```python
from build123d import *
from OCP.BRepFilletAPI import BRepFilletAPI_MakeChamfer

# Parameters (mm, degrees)
RESSALTO_EXTRUS_O2_DEPTH = 13
ESBO_O3_R                = 9.325
CORTE_EXTRUS_O1_DEPTH    = 27.211129951
ESBO_O4_W                = 8.746276247
ESBO_O4_H                = 4.85
CORTE_EXTRUS_O2_DEPTH    = 6.35
CHANFRO1_SIZE            = 2.5
CHANFRO1_SIZE2           = 1.443375673
CHANFRO2_SIZE            = 2
CHANFRO2_SIZE2           = 1.154700538
CHANFRO3_SIZE            = 2
CHANFRO3_SIZE2           = 1.154700538


with BuildPart() as part:
    # Esboço1 → Ressalto-extrusão2 (new body)
    with BuildSketch(Plane.XY):
        Polygon((0, 17.205038022), (-14.9, 8.602519011), (-14.9, -8.602519011), (0, -17.205038022), (14.9, -8.602519011), (14.9, 8.602519011), align=None)
    extrude(amount=RESSALTO_EXTRUS_O2_DEPTH)

    # Esboço3 → Corte-extrusão1 (cut, through all)
    with BuildSketch(Plane.XY.offset(13)):
        Circle(ESBO_O3_R)
    extrude(amount=-CORTE_EXTRUS_O1_DEPTH, mode=Mode.SUBTRACT)

    # Esboço4 → Corte-extrusão2 (cut)
    with BuildSketch(Plane.XY.offset(13)):
        with Locations((-10.526861876, 0)):
            Rectangle(ESBO_O4_W, ESBO_O4_H)
        Polygon((-5.349888396, 14.116278516), (-9.550111604, 11.691278516), (-5.176973481, 4.116781098), (-0.976750273, 6.541781098), align=None)
        Polygon((9.550111604, 11.691278516), (5.349888396, 14.116278516), (0.976750273, 6.541781098), (5.176973481, 4.116781098), align=None)
        with Locations((10.526861876, 0)):
            Rectangle(ESBO_O4_W, ESBO_O4_H)
        Polygon((5.349888396, -14.116278516), (9.550111604, -11.691278516), (5.176973481, -4.116781098), (0.976750273, -6.541781098), align=None)
        Polygon((-9.550111604, -11.691278516), (-5.349888396, -14.116278516), (-0.976750273, -6.541781098), (-5.176973481, -4.116781098), align=None)
    extrude(amount=-CORTE_EXTRUS_O2_DEPTH, mode=Mode.SUBTRACT)

    # Chanfro1: one chamfer whose edges measure the first distance from different faces: ONE call of the kernel's chamfer builder (chamfer() names one face for all edges)
    chanfro1_edges_1 = [part.edges().sort_by_distance(p)[0] for p in [
        (-14.9, 5.513759505, 13),
        (-14.9, -5.513759505, 13),
    ]]
    chanfro1_side_1 = [part.faces().sort_by_distance(p)[0] for p in [
        (-14.9, 0, 5.969058161),
    ]]
    chanfro1_edges_2 = [part.edges().sort_by_distance(p)[0] for p in [
        (-2.674944198, -15.660658269, 13),
        (-12.225055802, -10.146898764, 13),
    ]]
    chanfro1_side_2 = [part.faces().sort_by_distance(p)[0] for p in [
        (-7.45, -12.903778516, 5.969058161),
    ]]
    chanfro1_edges_3 = [part.edges().sort_by_distance(p)[0] for p in [
        (2.674944198, -15.660658269, 13),
        (12.225055802, -10.146898764, 13),
    ]]
    chanfro1_side_3 = [part.faces().sort_by_distance(p)[0] for p in [
        (7.45, -12.903778516, 5.969058161),
    ]]
    chanfro1_edges_4 = [part.edges().sort_by_distance(p)[0] for p in [
        (14.9, -5.513759505, 13),
        (14.9, 5.513759505, 13),
    ]]
    chanfro1_side_4 = [part.faces().sort_by_distance(p)[0] for p in [
        (14.9, 0, 5.969058161),
    ]]
    chanfro1_edges_5 = [part.edges().sort_by_distance(p)[0] for p in [
        (12.225055802, 10.146898764, 13),
        (2.674944198, 15.660658269, 13),
    ]]
    chanfro1_side_5 = [part.faces().sort_by_distance(p)[0] for p in [
        (7.45, 12.903778516, 5.969058161),
    ]]
    chanfro1_edges_6 = [part.edges().sort_by_distance(p)[0] for p in [
        (-12.225055802, 10.146898764, 13),
        (-2.674944198, 15.660658269, 13),
    ]]
    chanfro1_side_6 = [part.faces().sort_by_distance(p)[0] for p in [
        (-7.45, 12.903778516, 5.969058161),
    ]]
    chanfro1 = BRepFilletAPI_MakeChamfer(part.part.solid().wrapped)
    for e in chanfro1_edges_1:
        chanfro1.Add(CHANFRO1_SIZE, CHANFRO1_SIZE2, e.wrapped, chanfro1_side_1[0].wrapped)  # the first distance lies on this face
    for e in chanfro1_edges_2:
        chanfro1.Add(CHANFRO1_SIZE, CHANFRO1_SIZE2, e.wrapped, chanfro1_side_2[0].wrapped)  # the first distance lies on this face
    for e in chanfro1_edges_3:
        chanfro1.Add(CHANFRO1_SIZE, CHANFRO1_SIZE2, e.wrapped, chanfro1_side_3[0].wrapped)  # the first distance lies on this face
    for e in chanfro1_edges_4:
        chanfro1.Add(CHANFRO1_SIZE, CHANFRO1_SIZE2, e.wrapped, chanfro1_side_4[0].wrapped)  # the first distance lies on this face
    for e in chanfro1_edges_5:
        chanfro1.Add(CHANFRO1_SIZE, CHANFRO1_SIZE2, e.wrapped, chanfro1_side_5[0].wrapped)  # the first distance lies on this face
    for e in chanfro1_edges_6:
        chanfro1.Add(CHANFRO1_SIZE, CHANFRO1_SIZE2, e.wrapped, chanfro1_side_6[0].wrapped)  # the first distance lies on this face
    add(Compound.cast(chanfro1.Shape()), mode=Mode.REPLACE)

    # Chanfro2
    chanfro2_edges = [part.edges().sort_by_distance(p)[0] for p in [
        (-9.325, 0, 0),
    ]]
    chanfro2_side = [part.faces().sort_by_distance(p)[0] for p in [
        (-9.325, 0, 6.5),
    ]]
    chamfer(chanfro2_edges, length=CHANFRO2_SIZE, length2=CHANFRO2_SIZE2, reference=chanfro2_side[0])

    # Chanfro3
    chanfro3_edges = [part.edges().sort_by_distance(p)[0] for p in [
        (14.9, 0, 0),
        (7.45, -12.903778516, 0),
        (-7.45, -12.903778516, 0),
        (-14.9, 0, 0),
        (-7.45, 12.903778516, 0),
        (7.45, 12.903778516, 0),
    ]]
    chanfro3_side = [part.faces().sort_by_distance(p)[0] for p in [
        (-10.934903057, 0, 0),
    ]]
    chamfer(chanfro3_edges, length=CHANFRO3_SIZE, length2=CHANFRO3_SIZE2, reference=chanfro3_side[0])


solid = part.part
```
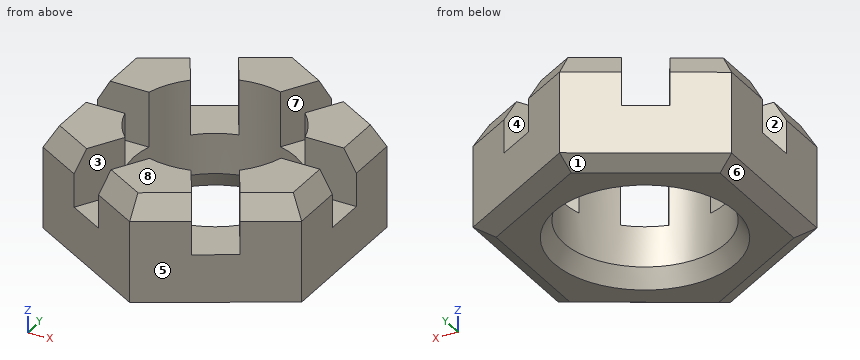
Work out the finished part from the listing and answer in its coordinate system (mm). Face numbers are marked on the shaded views. A direction names the side the tool comes from. Give positions to 0.01 mm unless a question says otherwise; leave off trailing zeros. Order: outer loops, then holes, each group sorted by start corner. A loop starts at its lowest first (then second) coordinate and runs counter-clockwise, first axis right, second up.
1. Section B-B, the plane y = 0 is taken. Determine the outline of the cut face in (x, z) (3 decimals).
Result sheet:
outline: (-14.9, 1.155) - (-12.9, 0) - (-10.48, 0) - (-9.325, 2) - (-9.325, 6.65) - (-14.9, 6.65) - close; (9.325, 2) - (10.48, 0) - (12.9, 0) - (14.9, 1.155) - (14.9, 6.65) - (9.325, 6.65) - close
2. Section D-D, the plane y = 11 is taken. Determine the outline of the cut face in (x, z), and give its area (3 significant figures).
Result sheet:
outline: (-10.75, 1.15) - (-6.75, 0) - (6.75, 0) - (10.75, 1.15) - (10.75, 10.5) - (9.15, 11.88) - (9.15, 6.65) - (3.55, 6.65) - (3.55, 13) - (-3.55, 13) - (-3.55, 6.65) - (-9.15, 6.65) - (-9.15, 11.88) - (-10.75, 10.5) - close
area: 198 mm2
3. Each of these flat-tipped pins is pushed along its axis until it touches: P1, Ø4.5, axis at x = -12, z = 11, coming from the +Y side; P2, Ø1.5, axis at x = -4.5, z = 4.5, coming from the +Y side; P3, Ø1.8, axis at x = 11, z = 10, coming from the -Y side; P4, Ø17, axis at x = 0, y = 0, coming from the +Z side. Where does it stop, or does it pass through?
Result sheet:
P1: stops at y = 11.54
P2: stops at y = 15.04
P3: stops at y = -11.37
P4: passes through
4. Section C-C, the plane z = 2.5 is taken. Determine the outline of the cut face in (x, y) (3 decimals).
Result sheet:
outline: (-14.9, -8.603) - (0, -17.205) - (14.9, -8.603) - (14.9, 8.603) - (0, 17.205) - (-14.9, 8.603) - close; hole circle Ø18.65 at (0, 0)
5. For the marked faces 1, 2, 3, 4 and 5, determine the directions among +Z, -Z, +X, -X, +Y, -Y from which every point of the face is accessible in a straight line to the end or side of a thin tool.
Result sheet:
face 1: -Z, -X, +Y
face 2: +Z, +X, -X
face 3: +Z, -Y
face 4: +Z, +Y
face 5: +Z, -Z, +X, -Y
6. The mould has two halves that part along X. Classify the marked faces 6, 7 and 8: released by +X, released by -X, zero draft, split by the parting line, or undercut.
Result sheet:
face 6: released by -X
face 7: undercut
face 8: zero draft
7. Straight lines are drawn through the part: L1, parallel to Y at x = 0.25, z = 10; L2, parallel to X at y = 3.5, z = 2.5; L3, parallel to X at y = -2.5, z = 0.5. For each, find the intervals that lie inside material, in ascending order.
Result sheet:
L1: y = -17.06 to -9.32, 9.32 to 17.06
L2: x = -14.9 to -8.64, 8.64 to 14.9
L3: x = -13.77 to -9.88, 9.88 to 13.77
8. Section A-A, the plane z = 9.5 is taken. Give the number of separate pieces and of enclosed holes in the cut face, and give its area (3 significant figures).
Result sheet:
separate pieces: 6
enclosed holes: 0
area: 331 mm2
